Here's how the part is built. I have some questions about the finished solid (model axes, mm). A direction names the side the tool comes from. Round coordinates to 2 decimals unless told otherwise and drop trailing zeros. Write each loop counter-clockwise with the first axis right and the second up, starting at its lowest first coordinate (ties: lowest second). Pieces come first, ordered by that corner, then holes. Notation, with made-up numbers: (52, -10) - (79, -10) arc R16 cw to (79, 9) - close; hole circle Ø5 at (80.25, 76). An arc over 180 degrees is marked (long way). One line per item, written item: value. Start each with the question number.
Item 1: If I drill on line 1 (X direction, y = 0.3, z = 12.5); line 2 (Y direction, x = -3.75, z = 3), over which ranges is the centre line in solid material (lowest first)?
Item 2: Imagine slicing it at D-D, the plane x = 3.25. Please give me the cut outline in (y, z).
Item 3: Imagine slicing it at B-B, the plane x = 0. Please give me the cut outline in (y, z).
Item 4: Thinking about a two-plate mould opening in Z: for faces 1 (the face through (0.1, 0.5, 9.5)), 2 (the face through (0, 0, 8)), 3 (the face through (-0.1, 0.5, 20)), which applies, released by +Z, released by -Z, zero draft, split by the parting line, or undercut?
Item 5: Imagine slicing it at A-A, the plane z = 12.5. Please give me the cut outline in (x, y).
Item 6: For faces 4 (the face through (0, 1, 9)), 5 (the face through (0, 9, 0)), which set-ups out of +Z, -Z, +X, -X, +Y, -Y let a thin tool reach every point of the face, with its end or its side?
Item 7: For P1, Ø3, axis at x = 3.5, z = 13, coming from the +Y side; P2, Ø6, axis at x = 3, y = 9, coming from the +Z side, each with a flat end and sliding along its axis, tell me the tip position at first contact or that it passes through.
```python
from build123d import *

# Parameters (mm, degrees)
ESQUISSE1_W             = 12
ESQUISSE1_H             = 20
ESQUISSE1_R             = 3
BOSS_EXTRU_1_DEPTH      = 1
ESQUISSE2_W             = 12
ESQUISSE2_H             = 1
BOSS_EXTRU_2_DEPTH      = 19
ESQUISSE3_R             = 3
ENL_V_MAT_EXTRU_1_DEPTH = 19
CONG_1_R                = 1
CONG_2_R                = 1


with BuildPart() as part:
    # Esquisse1 → Boss.-Extru.1 (new body)
    with BuildSketch(Plane.XY):
        with Locations((0, 10)):
            Rectangle(ESQUISSE1_W, ESQUISSE1_H)
        with Locations((0, 12.5)):
            Circle(ESQUISSE1_R, mode=Mode.SUBTRACT)
    extrude(amount=BOSS_EXTRU_1_DEPTH)

    # Esquisse2 → Boss.-Extru.2 (add)
    with BuildSketch(Plane.XY.offset(1)):
        with Locations((0, 0.5)):
            Rectangle(ESQUISSE2_W, ESQUISSE2_H)
    extrude(amount=BOSS_EXTRU_2_DEPTH)

    # Esquisse3 → Enlèv. mat.-Extru.1 (cut)
    with BuildSketch(Plane(origin=(0, 1, 0), x_dir=(1, 0, 0), z_dir=(0, 1, 0))):
        with Locations(Location((0, -12.5, 0), (0, 0, 270))):
            Circle(ESQUISSE3_R)
    extrude(amount=-ENL_V_MAT_EXTRU_1_DEPTH, mode=Mode.SUBTRACT)

    # Congé1
    cong_1_edges = [part.edges().sort_by_distance(p)[0] for p in [
        (0, 1, 1),
        (0, 0, 0),
    ]]
    fillet(cong_1_edges, radius=CONG_1_R)

    # Congé2
    cong_2_edges = [part.edges().sort_by_distance(p)[0] for p in [
        (-6, 0.5, 20),
        (6, 0.5, 20),
        (-6, 20, 0.5),
        (6, 20, 0.5),
    ]]
    fillet(cong_2_edges, radius=CONG_2_R)


solid = part.part
```
Values follow:
1. line 1: x = -6 to -3, 3 to 6
1. line 2: y = 0 to 1
2. outline: (0, 1) arc R1 ccw to (1, 0) - (20, 0) - (20, 1) - (2, 1) arc R1 cw to (1, 2) - (1, 20) - (0, 20) - close
3. outline: (0, 1) arc R1 ccw to (1, 0) - (9.5, 0) - (9.5, 1) - (2, 1) arc R1 cw to (1, 2) - (1, 9.5) - (0, 9.5) - close; (0, 15.5) - (1, 15.5) - (1, 20) - (0, 20) - close; (15.5, 0) - (20, 0) - (20, 1) - (15.5, 1) - close
4. face 1: undercut
4. face 2: zero draft
4. face 3: released by +Z
5. outline: (-6, 0) - (-3, 0) - (-3, 1) - (-6, 1) - close; (3, 0) - (6, 0) - (6, 1) - (3, 1) - close
6. face 4: +Z, +X, -X, +Y
6. face 5: -Z, +X, -X, +Y, -Y
7. P1: stops at y = 1
7. P2: stops at z = 1
